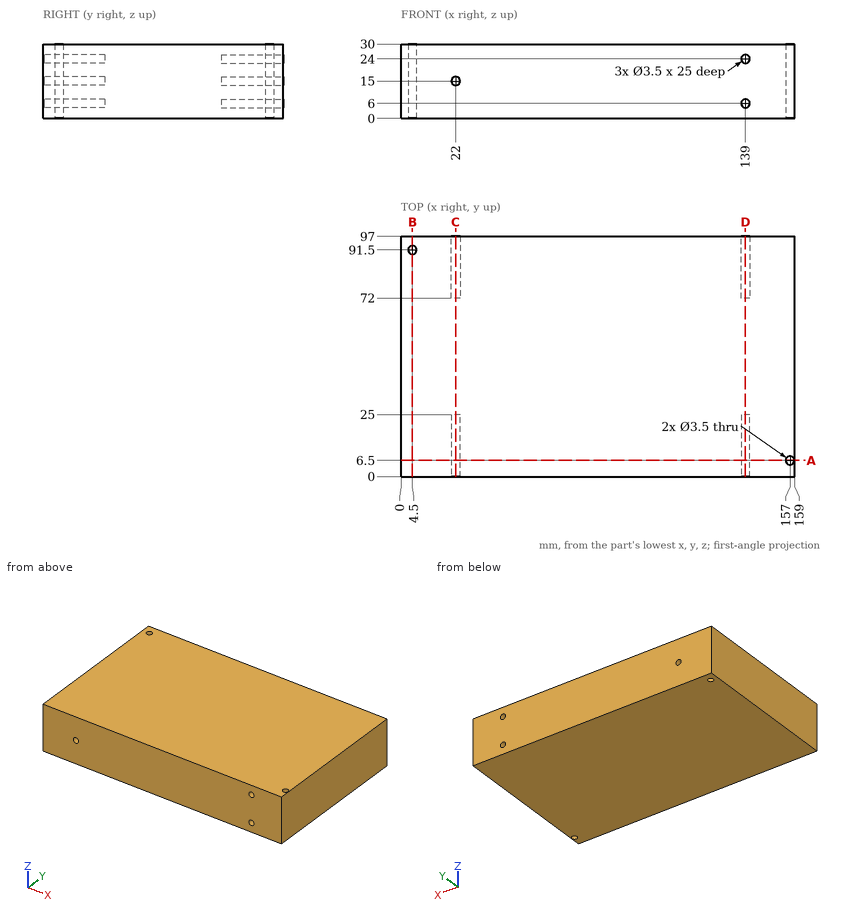
The drawing under review shows one solid part. Ordinate dimensions are in mm from its lowest x, y, z. Round coordinates to 2 decimals unless told otherwise and drop trailing zeros. Order: outer loops, then holes, each group sorted by start corner. A loop starts at its lowest first (then second) coordinate and runs counter-clockwise, first axis right, second up. Notation, with made-up numbers: (40.5, 15.5) -> (69.5, 15.5) arc R35 ccw to (69.5, 54.5) -> close; hole circle Ø3 at (55, -8.5). An arc over 180 degrees is marked (long way). Use a Markdown table: item, result.
Item 1: Take a section at B-B (x = 4.5). State the section outline as (y, z) points.
Resolved:
| item | result |
|---|---|
| outline | (0, 0) -> (89.75, 0) -> (89.75, 30) -> (0, 30) -> close; (93.25, 0) -> (97, 0) -> (97, 30) -> (93.25, 30) -> close |
Item 2: Take a section at D-D (x = 139). State the section outline as (y, z) points.
Resolved:
| item | result |
|---|---|
| outline | (0, 0) -> (97, 0) -> (97, 4.25) -> (72, 4.25) -> (72, 7.75) -> (97, 7.75) -> (97, 22.25) -> (72, 22.25) -> (72, 25.75) -> (97, 25.75) -> (97, 30) -> (0, 30) -> (0, 25.75) -> (25, 25.75) -> (25, 22.25) -> (0, 22.25) -> (0, 7.75) -> (25, 7.75) -> (25, 4.25) -> (0, 4.25) -> close |
Item 3: Take a section at A-A (y = 6.5). State the section outline as (x, z) points.
Resolved:
| item | result |
|---|---|
| outline | (0, 0) -> (155.25, 0) -> (155.25, 30) -> (0, 30) -> close; (158.75, 0) -> (159, 0) -> (159, 30) -> (158.75, 30) -> close; hole circle Ø3.5 at (22, 15); hole circle Ø3.5 at (139, 6); hole circle Ø3.5 at (139, 24) |
Item 4: For line 1 along Z through (x, y) = (22, 11.75); line 2 along X through (y, z) = (12, 16), list the stretches that pass through material, from the lowest coordinate up. Write a range as [from, to].
Resolved:
| item | result |
|---|---|
| line 1 | z = [0, 13.25], [16.75, 30] |
| line 2 | x = [0, 20.56], [23.44, 159] |
Item 5: For pin 1 (3 mm diameter, centred on x = 22, z = 15, fed in from -Y); pin 2 (2 mm diameter, centred on x = 157, y = 6.5, fed in from -Z); pin 3 (1 mm diameter, centred on x = 138.5, z = 6, fed in from +Y), all flat-tipped, find the tip position at first contact; note any pin that passes through.
Resolved:
| item | result |
|---|---|
| pin 1 | stops at y = 25 |
| pin 2 | passes through |
| pin 3 | stops at y = 72 |
Item 6: Take a section at C-C (x = 22). State the section outline as (y, z) points.
Resolved:
| item | result |
|---|---|
| outline | (0, 0) -> (97, 0) -> (97, 13.25) -> (72, 13.25) -> (72, 16.75) -> (97, 16.75) -> (97, 30) -> (0, 30) -> (0, 16.75) -> (25, 16.75) -> (25, 13.25) -> (0, 13.25) -> close |
